Build history of the part. All positions in model axes, mm. A direction names the side the tool comes from. Round coordinates to 2 decimals unless told otherwise and drop trailing zeros. Loops run counter-clockwise (first coordinate to the right, second up) from the corner with the lowest first, then second, coordinate; pieces in that order, holes last. Notation, with made-up numbers: (19.5, 72) -> (28.5, 72) arc R20 ccw to (28.5, 81) -> close; hole circle Ø3 at (9.5, 33). An arc over 180 degrees is marked (long way). Put each result on its own line as item: value. Start each with the question number.
Item 1: Drill centre lines: probe 1 along Z at (x, y) = (1.5, 71); probe 2 along Z at (x, y) = (-9, 29.5); probe 3 along X at (y, z) = (54.5, 97.5). Where is each one in solid material? Low to high. Write a range as [from, to].
Item 2: Cut at B-B, the plane x = -22.5. List the corners of the cut face in (y, z).
Item 3: Cut at C-C, the plane z = 113. List the corners of the cut face in (x, y), plus the area to 3 significant figures.
Item 4: Cut at D-D, the plane x = -11. List the corners of the cut face in (y, z), plus the area to 3 significant figures.
Item 5: Cut at A-A, the plane y = 62. List the corners of the cut face in (x, z), plus the area to 3 significant figures.
Item 6: Tool access for faces 4 (the flat face through (-1, 0, 114)), 5 (the flat face through (16.267, 50, 129)), 6 (the cylindrical face through (0.228, 18.286, 117.475)), 7 (the flat face through (-16.267, 50, 128)), 8 (the cylindrical face through (26.834, 73.935, 145.771)): list every direction of +Z, -Z, +X, -X, +Y, -Y with a clear straight run to the whole face (end or side of a thin tool).
Item 7: Flat gauge pins, fed straight in: pin 1 Ø6.5 at (x, y) = (-28.01, 76.2) entering from +Z; pin 2 Ø19 at (x, y) = (33, 28.5) entering from -Z; pin 3 Ø14.5 at (y, z) = (28, 113.5) entering from +X; pin 4 Ø24 at (y, z) = (26, 128.5) entering from -X. Where does each tip first touch, or does it go through?
Item 8: Pull direction Z, two halves, no side cores. Call faces 1 (the cylindrical face through (0.228, 81.783, 117.754)), 2 (the cylindrical face through (-29.19, 73.935, 145.771)), 3 (the cylindrical face through (0.58, 50.09, 88.9)): +Z half, -Z half, draft (parallel to the pull), parting line (faces both ways), or undercut.
```python
from build123d import *

# Parameters (mm, degrees)
BOSS_EXTRUDE1_DEPTH         = 101.6
CUT_EXTRUDE1_DEPTH          = 57.023894283
TAP_DRILL_FOR_1_4_20_TAP2_D = 5.1054


with BuildPart() as part:
    # Sketch1 → Boss-Extrude1 (new body)
    with BuildSketch(Plane(origin=(0, 0, 0), x_dir=(1, 0, 0), z_dir=(0, 1, 0))):
        with BuildLine():
            Line((-16.266605643, -141.378421793), (-39.75728864, -141.378421793))
            Line((-39.75728864, -141.378421793), (-39.75728864, -150.287727069))
            Line((-39.75728864, -150.287727069), (39.75728864, -150.287727069))
            Line((39.75728864, -150.287727069), (39.75728864, -141.378421793))
            Line((39.75728864, -141.378421793), (16.266605643, -141.378421793))
            Line((16.266605643, -141.378421793), (16.266605643, -93.850732767))
            ThreePointArc((16.266605643, -93.850732767), (28.248414097, -90.964771208), (39.75728864, -86.555880794))
            Line((39.75728864, -86.555880794), (39.75728864, -79.51457728))
            ThreePointArc((39.75728864, -79.51457728), (0, -88.9), (-39.75728864, -79.51457728))
            Line((-39.75728864, -79.51457728), (-39.75728864, -86.555880794))
            ThreePointArc((-39.75728864, -86.555880794), (-28.248414097, -90.964771208), (-16.266605643, -93.850732767))
            Line((-16.266605643, -93.850732767), (-16.266605643, -141.378421793))
        make_face()
    extrude(amount=BOSS_EXTRUDE1_DEPTH)

    # Sketch2 → Cut-Extrude1 (cut, through all)
    with BuildSketch(Plane(origin=(16.266605643, 0, 0), x_dir=(0, 0, -1), z_dir=(1, 0, 0))):
        with BuildLine():
            Line((-111.26457728, 75.434320996), (-111.26457728, 24.634320996))
            ThreePointArc((-111.26457728, 24.634320996), (-117.61457728, 18.284320996), (-123.96457728, 24.634320996))
            Line((-123.96457728, 24.634320996), (-123.96457728, 75.434320996))
            ThreePointArc((-123.96457728, 75.434320996), (-117.61457728, 81.784320996), (-111.26457728, 75.434320996))
        make_face()
    extrude(amount=-CUT_EXTRUDE1_DEPTH, mode=Mode.SUBTRACT)

    # Tap Drill for 1/4-20 Tap2 (through all)
    with Locations(Plane.XY.offset(150.287727069)):
        with Locations((28.011947142, 76.2), (-28.011947142, 76.2), (-28.011947142, 25.4), (28.011947142, 25.4)):
            Hole(TAP_DRILL_FOR_1_4_20_TAP2_D / 2)


solid = part.part
```
Reply:
1. probe 1: z = [88.89, 111.26], [123.96, 150.29]
1. probe 2: z = [88.44, 111.26], [123.96, 150.29]
1. probe 3: x = [-16.27, 16.27]
2. outline: (0, 86.01) -> (101.6, 86.01) -> (101.6, 92.55) -> (0, 92.55) -> close; (0, 141.38) -> (101.6, 141.38) -> (101.6, 150.29) -> (0, 150.29) -> close
3. outline: (-16.27, 0) -> (16.27, 0) -> (16.27, 20.27) -> (-16.27, 20.27) -> close; (-16.27, 79.8) -> (16.27, 79.8) -> (16.27, 101.6) -> (-16.27, 101.6) -> close
3. area: 1,370 mm^2
4. outline: (0, 88.22) -> (101.6, 88.22) -> (101.6, 150.29) -> (0, 150.29) -> close; hole (24.63, 111.26) -> (75.43, 111.26) arc R6.35 ccw to (75.43, 123.96) -> (24.63, 123.96) arc R6.35 ccw to start
4. area: 5,530 mm^2
5. outline: (-39.76, 79.51) arc R88.9 cw to (39.76, 79.51) -> (39.76, 86.56) arc R95.25 ccw to (16.27, 93.85) -> (16.27, 111.26) -> (-16.27, 111.26) -> (-16.27, 93.85) arc R95.25 ccw to (-39.76, 86.56) -> close; (-39.76, 141.38) -> (-16.27, 141.38) -> (-16.27, 123.96) -> (16.27, 123.96) -> (16.27, 141.38) -> (39.76, 141.38) -> (39.76, 150.29) -> (-39.76, 150.29) -> close
5. area: 2,330 mm^2
6. face 4: +Z, -Z, +X, -X, -Y
6. face 5: +X, +Y, -Y
6. face 6: +X, -X
6. face 7: -X, +Y, -Y
6. face 8: +Z, -Z
7. pin 1: stops at z = 150.29
7. pin 2: stops at z = 79.51
7. pin 3: stops at x = 16.27
7. pin 4: stops at x = -16.27
8. face 1: undercut
8. face 2: draft
8. face 3: -Z half
